from build123d import *

# Parameters (mm, degrees)
SKETCH_2_W               = 50
SKETCH_2_H               = 50
EXTRUDE_1_DEPTH          = 100
EXTRUDE_1_TAPER          = 10
SKETCH_3_W               = 215.720321278
SKETCH_3_H               = 290.879799434
CUT_EXTRUDE_1_DEPTH      = 107.066017319
SKETCH_7_W               = 4.5
SKETCH_7_H               = 23.792731937
SKETCH_8_W               = 50
SKETCH_8_H               = 4.5
CUT_EXTRUDE_2_DEPTH      = 9
SKETCH_9_W               = 9
SKETCH_9_H               = 9
CUT_EXTRUDE_3_DEPTH      = 4.5
SKETCH_10_W              = 7
SKETCH_10_H              = 3.5
CUT_EXTRUDE_4_DEPTH      = 10.5
SKETCH_11_R              = 2.25
CUT_EXTRUDE_5_DEPTH      = 20
CUT_EXTRUDE_6_DEPTH      = 107.066017319
CUT_EXTRUDE_6_DEPTH_BACK = 107.066017319
SKETCH_12_W              = 75.055418853
SKETCH_12_H              = 23.361905794


with BuildPart() as part:
    # 草圖2 → 填料-伸長1 (new body)
    with BuildSketch(Plane(origin=(0, 0, 0), x_dir=(1, 0, 0), z_dir=(0, 1, 0))):
        Rectangle(SKETCH_2_W, SKETCH_2_H)
    extrude(amount=EXTRUDE_1_DEPTH, taper=EXTRUDE_1_TAPER)

    # 草圖3 → 除料-伸長1 (cut, through all)
    with BuildSketch(Plane.XY):
        Rectangle(SKETCH_3_W, SKETCH_3_H)
    extrude(amount=CUT_EXTRUDE_1_DEPTH, mode=Mode.SUBTRACT)


with BuildPart() as body_2:
    # stick_antenna_434MHz: read off the stored shape, not the designer's step
    # stick_antenna_434MHz outline → stick_antenna_434MHz (revolve)
    with BuildSketch(Plane.XY):
        Polygon((0, 94.2), (0, 23), (3, 23), (3, 18), (6.4, 18), (6.4, 35.2), (5, 62.2), (5, 81.2), (5.5, 81.2), (6, 82.2), (6, 94.2), align=None)
    revolve(axis=Axis((0, 0, 0), (0, 1, 0)))


with BuildPart() as part_1:
    add(part.part)

    # Other 1: read off the stored shape, not the designer's step
    # Other 1: cut body 2
    add(body_2.part, mode=Mode.SUBTRACT)

    # 草圖7 → 除料-旋轉1 (revolve, cut)
    with BuildSketch(Plane.XY):
        with Locations((2.25, 11.896365969)):
            Rectangle(SKETCH_7_W, SKETCH_7_H)
    revolve(axis=Axis((0, 30.263839144, 0), (0, -1, 0)), mode=Mode.SUBTRACT)

    # 草圖8 → 除料-伸長2 (cut)
    with BuildSketch(Plane.XZ):
        with Locations((0, -2.25)):
            Rectangle(SKETCH_8_W, SKETCH_8_H)
    extrude(amount=-CUT_EXTRUDE_2_DEPTH, mode=Mode.SUBTRACT)

    # 草圖9 → 除料-伸長3 (cut)
    with BuildSketch(Plane.XY):
        with Locations((0, 13.5)):
            Rectangle(SKETCH_9_W, SKETCH_9_H)
    extrude(amount=-CUT_EXTRUDE_3_DEPTH, mode=Mode.SUBTRACT)

    # 草圖10 → 除料-伸長4 (cut)
    with BuildSketch(Plane.XY.offset(-25)):
        with Locations((-18, 21.75)):
            Rectangle(SKETCH_10_W, SKETCH_10_H)
    cut_extrude_4 = extrude(amount=CUT_EXTRUDE_4_DEPTH, mode=Mode.SUBTRACT)

    # 草圖11 → 除料-伸長5 (cut)
    with BuildSketch(Plane.XZ):
        with Locations(Location((-18, -18, 0), (0, 0, 270))):
            Circle(SKETCH_11_R)
        with Locations(Location((18, -18, 0), (0, 0, 90))):
            Circle(SKETCH_11_R)
    extrude(amount=-CUT_EXTRUDE_5_DEPTH, mode=Mode.SUBTRACT)

    # 鏡射2: 除料-伸長4 across plane
    add(cut_extrude_4.mirror(Plane(origin=(0, 0, 0), x_dir=(0, 0, 1), z_dir=(1, 0, 0))), mode=Mode.SUBTRACT)

    # 草圖12 → 除料-伸長6 (cut, two sides: drawn at the far end of the back side and taken through both)
    with BuildSketch(Plane(origin=(0, 0, 0), x_dir=(0, 0, -1), z_dir=(1, 0, 0)).offset(-CUT_EXTRUDE_6_DEPTH_BACK)):
        with Locations((61.527709427, 0)):
            Rectangle(SKETCH_12_W, SKETCH_12_H)
    extrude(amount=CUT_EXTRUDE_6_DEPTH + CUT_EXTRUDE_6_DEPTH_BACK, mode=Mode.SUBTRACT)


solid = part_1.part
Verification items for the finished model (mm, model axes). A direction names the side the tool comes from. Give positions to 0.01 mm unless a question says otherwise; leave off trailing zeros. Write item = value, one per line. Start each with the question number.
Q1. Depth check by flat-ended pin: P1, Ø1.9, axis at x = -17, z = -17.5, coming from the -Y side; P2, Ø1.1, axis at x = 18, y = 22, coming from the -Z side; P3, Ø8, axis at x = -11, y = 30.5, coming from the -Z side. Enter the tip coordinate at first touch or a pass-through.
Q2. Tool access check on faces 4 (the face through (-18, 22, -14.5)), 5 (the face through (18, 23.5, -18)), 6 (the face through (4.5, 13, -2)), 7 (the face through (0, 94.2, -2)), 8 (the face through (14, 9, -2)). Record the directions out of +Z, -Z, +X, -X, +Y, -Y that give a thin tool (end or side, any length) a straight path to the whole face; none if there is none.
Q3. Mould release check, pull along X, two halves, no side actions. Record for faces 1 (the face through (0, 88, -6)), 2 (the face through (0, 3, -24)), 3 (the face through (14.5, 22, -18)): released by +X, released by -X, zero draft, split by the parting line, or undercut.
Q4. Thickness scan on line 1 (X direction, y = 11.5, z = -18); line 2 (X direction, y = 15.25, z = -18); line 3 (Z direction, x = 16.5, y = 14.5). Record the ranges inside material, lowest first.
Q5. Cross-section at A-A, the plane z = -18. State how many separate pieces and enclosed holes the cut face has, and give its area (3 significant figures).
Answer key:
q1.P1 = 23.5
q1.P2 = -14.5
q1.P3 = -20.33
q2.face_4 = -Z, -X
q2.face_5 = -Z, +X
q2.face_6 = +Z, -Y
q2.face_7 = +Z
q2.face_8 = +Z, +X, -X, -Y
q3.face_1 = undercut
q3.face_2 = zero draft
q3.face_3 = released by +X
q4.line_1 = -22.97 to -20.25, -15.75 to 15.75, 20.25 to 22.97
q4.line_2 = -22.31 to -20.25, -15.75 to 15.75, 20.25 to 22.31
q4.line_3 = -22.44 to -19.68, -16.32 to 0
q5.separate_pieces = 3
q5.enclosed_holes = 0
q5.area = 1,480 mm^2
